```python
from build123d import *


with BuildPart() as f2:
    # F0 (on Right) → F2 (revolve)
    with BuildSketch(Plane.YZ):
        with BuildLine():
            Line((-52.6758568757, 24.765), (-59.055, 21.082))
            Line((-59.055, 21.082), (-20.955, 21.082))
            Line((-20.955, 21.082), (-20.955, 15.875))
            Line((-20.955, 15.875), (0, 15.875))
            ThreePointArc((0, 15.875), (11.2253201513, 11.2253201513), (15.875, 0))
            Line((15.875, 0), (24.765, 0))
            ThreePointArc((24.765, 0), (17.5114994361, 17.5114994361), (0, 24.765))
            Line((0, 24.765), (-52.6758568757, 24.765))
        make_face()
        with BuildLine():
            Line((-20.955, 21.082), (-59.055, 21.082))
            Line((-59.055, 21.082), (-59.055, 0))
            Line((-59.055, 0), (0, 0))
            Line((0, 0), (10.5189766587, 0))
            Line((10.5189766587, 0), (15.875, 0))
            ThreePointArc((15.875, 0), (11.2253201513, 11.2253201513), (0, 15.875))
            Line((0, 15.875), (-20.955, 15.875))
            Line((-20.955, 15.875), (-20.955, 21.082))
        make_face()
    revolve(axis=Axis((0, -21.59, 0), (0, 1, 0)))

    # F1 (on Right) → F3 (revolve)
    with BuildSketch(Plane.YZ):
        with BuildLine():
            Line((-24.765, -52.6758568757), (-21.082, -59.055))
            Line((-21.082, -59.055), (-21.082, -20.955))
            Line((-21.082, -20.955), (-15.875, -20.955))
            Line((-15.875, -20.955), (-15.875, 0))
            ThreePointArc((-15.875, 0), (-11.2253201513, 11.2253201513), (0, 15.875))
            Line((0, 15.875), (0, 24.765))
            ThreePointArc((0, 24.765), (-17.5114994361, 17.5114994361), (-24.765, 0))
            Line((-24.765, 0), (-24.765, -52.6758568757))
        make_face()
        with BuildLine():
            Line((-21.082, -20.955), (-21.082, -59.055))
            Line((-21.082, -59.055), (0, -59.055))
            Line((0, -59.055), (0, 0))
            Line((0, 0), (0, 15.875))
            ThreePointArc((0, 15.875), (-11.2253201513, 11.2253201513), (-15.875, 0))
            Line((-15.875, 0), (-15.875, -20.955))
            Line((-15.875, -20.955), (-21.082, -20.955))
        make_face()
    revolve(axis=Axis((0, 0, -21.59), (0, 0, 1)))

    # F0 (on Right) → F4 (revolve, cut)
    with BuildSketch(Plane.YZ):
        with BuildLine():
            Line((-20.955, 21.082), (-59.055, 21.082))
            Line((-59.055, 21.082), (-59.055, 0))
            Line((-59.055, 0), (0, 0))
            Line((0, 0), (10.5189766587, 0))
            Line((10.5189766587, 0), (15.875, 0))
            ThreePointArc((15.875, 0), (11.2253201513, 11.2253201513), (0, 15.875))
            Line((0, 15.875), (-20.955, 15.875))
            Line((-20.955, 15.875), (-20.955, 21.082))
        make_face()
    revolve(axis=Axis((0, -21.59, 0), (0, 1, 0)), mode=Mode.SUBTRACT)

    # F1 (on Right) → F5 (revolve, cut)
    with BuildSketch(Plane.YZ):
        with BuildLine():
            Line((-21.082, -20.955), (-21.082, -59.055))
            Line((-21.082, -59.055), (0, -59.055))
            Line((0, -59.055), (0, 0))
            Line((0, 0), (0, 15.875))
            ThreePointArc((0, 15.875), (-11.2253201513, 11.2253201513), (-15.875, 0))
            Line((-15.875, 0), (-15.875, -20.955))
            Line((-15.875, -20.955), (-21.082, -20.955))
        make_face()
    revolve(axis=Axis((0, 0, -21.59), (0, 0, 1)), mode=Mode.SUBTRACT)


solid = f2.part
```
For this review, take the finished solid that the model builds, in its own axes (mm). A direction names the side the tool comes from. Coordinates: 2 decimals unless noted, no trailing zeros. Loops run counter-clockwise (first coordinate to the right, second up) from the corner with the lowest first, then second, coordinate; pieces in that order, holes last. Notation, with made-up numbers: (-15, -10) -> (8, -10) arc R18 ccw to (8, 4) -> close; hole circle Ø7 at (71.25, -8.75). An arc over 180 degrees is marked (long way). Return JSON: item names as keys, results as strings. Group by question number.
(1) Consider section B-B, the plane y = -38.5. Give the boundary of the cut face in (x, z) (3 decimals), plus the area to 3 significant figures.
(2) Tool access review of faces 1 (the cylindrical face through (1.09, 24.74, -26.71)), 2 (the cylindrical face through (4.77, -12.95, 15.14)): name each direction out of +Z, -Z, +X, -X, +Y, -Y from which nothing blocks a thin tool from reaching the whole face with its end or side.
(3) Consider section A-A, the plane x = 0. Give the boundary of the cut face in (y, z) (3 decimals).
(4) To check wall thickness, follow L1, parallel to X at y = -30, z = 0 (3 decimals); L2, parallel to X at y = -0.5, z = -10. State the ranges of each line that lie inside material, in increasing order.
(5) Mouldability with a two-part tool opening along X and no side actions: class faces 3 (the conical face through (-20.755, 4.609, -58.745)), 4 (the cylindrical face through (6.33, -20.11, -40.27)) as pulls with the +X half, pulls with the -X half, needs draft (parallel to the pull), parting line crosses it, or undercut.
(6) For pin 1 Ø21 at (x, y) = (-3, 6) entering from -Z (3 decimals); pin 2 Ø12 at (x, z) = (-8.5, -13) entering from +Y; pin 3 Ø12 at (y, z) = (8.5, -42.5) entering from -X, all flat-tipped, find the tip position at first contact; note any pin that passes through.
Results below:
{
 "1": {"outline": "circle Ø49.53 at (0, 0); hole circle Ø42.164 at (0, 0)", "area": "530 mm2"},
 "2": {"face 1": "-Z", "face 2": "-Y"},
 "3": {"outline": "(-59.055, -21.082) -> (-52.676, -24.765) -> (-24.765, -24.765) -> (-24.765, -52.676) -> (-21.082, -59.055) -> (-21.082, -21.082) -> close; (-59.055, 21.082) -> (-20.955, 21.082) -> (-20.955, 15.875) -> (0, 15.875) arc R15.875 cw to (15.875, 0) -> (15.875, -20.955) -> (21.082, -20.955) -> (21.082, -59.055) -> (24.765, -52.676) -> (24.765, 0) arc R24.765 ccw to (0, 24.765) -> (-52.676, 24.765) -> close; (-20.955, -20.955) -> (-15.875, -20.955) -> (-15.875, -15.875) -> (-20.955, -15.875) -> close"},
 "4": {"L1": "x = -24.765 to -21.082, 21.082 to 24.765", "L2": "x = -24.76 to -15.87, 15.87 to 24.76"},
 "5": {"face 3": "parting line crosses it", "face 4": "undercut"},
 "6": {"pin 1": "stops at z = -20.955", "pin 2": "stops at y = 24.64", "pin 3": "stops at x = -24.64"}
}
